from build123d import *

# Parameters (mm, degrees)
SKETCH_1_W       = 16
SKETCH_1_H       = 16
EXTRUDE_1_DEPTH  = 4
SKETCH_2_R       = 6.5
EXTRUDE_2_DEPTH  = 7
SKETCH_3_R       = 6
EXTRUDE_3_DEPTH  = 12
EXTRUDE_START    = -2
SKETCH_4_R       = 6.5
EXTRUDE_4_DEPTH  = 2
SKETCH_6_R       = 1
EXTRUDE_5_DEPTH  = 3.6
SKETCH_7_W       = 26
SKETCH_7_H       = 27
EXTRUDE_6_DEPTH  = 1.5
SKETCH_8_W       = 10
SKETCH_8_H       = 22
EXTRUDE_7_DEPTH  = 4
SKETCH_9_R       = 0.6
EXTRUDE_8_DEPTH  = 4
SKETCH_10_R      = 0.6
EXTRUDE_9_DEPTH  = 1.5
SKETCH_11_W      = 4.148660329
SKETCH_11_H      = 3.0926377
EXTRUDE_10_DEPTH = 1.5


with BuildPart() as part:
    # 草图1 → 凸台-拉伸1 (new body)
    with BuildSketch(Plane.XY):
        Rectangle(SKETCH_1_W, SKETCH_1_H)
    extrude(amount=EXTRUDE_1_DEPTH)

    # 草图2 → 凸台-拉伸2 (add)
    with BuildSketch(Plane.XY.offset(4)):
        with Locations(Location((0, 0, 0), (0, 0, 180))):
            Circle(SKETCH_2_R)
    extrude(amount=EXTRUDE_2_DEPTH)

    # 草图3 → 凸台-拉伸3 (add)
    with BuildSketch(Plane.XY.offset(11)):
        Circle(SKETCH_3_R)
    extrude(amount=EXTRUDE_3_DEPTH)

    # 草图4 → 凸台-拉伸4 (add)
    with BuildSketch(Plane.XY.offset(23).offset(EXTRUDE_START)):
        with Locations(Location((0, 0, 0), (0, 0, 180))):
            Circle(SKETCH_4_R)
    extrude(amount=EXTRUDE_4_DEPTH)

    # 草图5 → 切除-旋转2 (revolve, cut)
    with BuildSketch(Plane.XY.offset(23)):
        with BuildLine():
            Line((0, 2), (0, -2))
            ThreePointArc((0, -2), (2, 0), (0, 2))
        make_face()
    revolve(axis=Axis((0, 2, 23), (0, -1, 0)), mode=Mode.SUBTRACT)

    # 草图6 → 凸台-拉伸5 (add)
    # profile 1 of 2: a face of its own
    with BuildSketch(Plane(origin=(0, 0, 0), x_dir=(-1, 0, 0), z_dir=(0, 0, -1))):
        with BuildLine():
            Line((-1.8, 8), (-1.8, 11.5))
            ThreePointArc((-1.8, 11.5), (0, 13.3), (1.8, 11.5))
            Line((1.8, 11.5), (1.8, 8))
            Line((1.8, 8), (-1.8, 8))
        make_face()
        with Locations((0, 11.5)):
            Circle(SKETCH_6_R, mode=Mode.SUBTRACT)
    # profile 2 of 2: a face of its own
    with BuildSketch(Plane(origin=(0, 0, 0), x_dir=(-1, 0, 0), z_dir=(0, 0, -1))):
        with BuildLine():
            Line((-1.8, -8), (1.8, -8))
            Line((1.8, -8), (1.8, -11.5))
            ThreePointArc((1.8, -11.5), (0, -13.3), (-1.8, -11.5))
            Line((-1.8, -11.5), (-1.8, -8))
        make_face()
        with Locations(Location((0, -11.5, 0), (0, 0, 180))):
            Circle(SKETCH_6_R, mode=Mode.SUBTRACT)
    extrude(amount=-EXTRUDE_5_DEPTH)

    # 草图7 → 凸台-拉伸6 (add)
    with BuildSketch(Plane(origin=(0, 0, 0), x_dir=(-1, 0, 0), z_dir=(0, 0, -1))):
        with Locations((4, 0)):
            Rectangle(SKETCH_7_W, SKETCH_7_H)
    extrude(amount=EXTRUDE_6_DEPTH)

    # 草图8 → 凸台-拉伸7 (add)
    with BuildSketch(Plane(origin=(0, 0, -1.5), x_dir=(-1, 0, 0), z_dir=(0, 0, -1))):
        with Locations((16, 0)):
            Rectangle(SKETCH_8_W, SKETCH_8_H)
    extrude(amount=EXTRUDE_7_DEPTH)

    # 草图9 → 凸台-拉伸8 (add)
    with BuildSketch(Plane.ZY.offset(21)):
        with Locations(Location((-3.5, 0, 0), (0, 0, 180))):
            Circle(SKETCH_9_R)
        with Locations(Location((-3.5, 3, 0), (0, 0, 180))):
            Circle(SKETCH_9_R)
        with Locations(Location((-3.5, 6, 0), (0, 0, 180))):
            Circle(SKETCH_9_R)
        with Locations(Location((-3.5, 9, 0), (0, 0, 180))):
            Circle(SKETCH_9_R)
        with Locations(Location((-3.5, -9, 0), (0, 0, 180))):
            Circle(SKETCH_9_R)
        with Locations(Location((-3.5, -6, 0), (0, 0, 180))):
            Circle(SKETCH_9_R)
        with Locations(Location((-3.5, -3, 0), (0, 0, 180))):
            Circle(SKETCH_9_R)
    extrude(amount=EXTRUDE_8_DEPTH)

    # 草图10 → 凸台-拉伸9 (add)
    with BuildSketch(Plane.XY):
        with Locations(Location((-12, 9, 0), (0, 0, 180))):
            Circle(SKETCH_10_R)
        with Locations(Location((-15, 9, 0), (0, 0, 180))):
            Circle(SKETCH_10_R)
        with Locations(Location((-15, 6, 0), (0, 0, 180))):
            Circle(SKETCH_10_R)
        with Locations(Location((-15, 3, 0), (0, 0, 180))):
            Circle(SKETCH_10_R)
        with Locations(Location((-15, 0, 0), (0, 0, 180))):
            Circle(SKETCH_10_R)
        with Locations(Location((-15, -3, 0), (0, 0, 180))):
            Circle(SKETCH_10_R)
        with Locations(Location((-15, -6, 0), (0, 0, 180))):
            Circle(SKETCH_10_R)
        with Locations(Location((-15, -9, 0), (0, 0, 180))):
            Circle(SKETCH_10_R)
        with Locations(Location((-12, 6, 0), (0, 0, 180))):
            Circle(SKETCH_10_R)
        with Locations(Location((-12, 3, 0), (0, 0, 180))):
            Circle(SKETCH_10_R)
        with Locations(Location((-12, 0, 0), (0, 0, 180))):
            Circle(SKETCH_10_R)
        with Locations(Location((-12, -3, 0), (0, 0, 180))):
            Circle(SKETCH_10_R)
        with Locations(Location((-12, -6, 0), (0, 0, 180))):
            Circle(SKETCH_10_R)
        with Locations(Location((-12, -9, 0), (0, 0, 180))):
            Circle(SKETCH_10_R)
    extrude(amount=EXTRUDE_9_DEPTH)

    # 草图11 → 凸台-拉伸10 (add)
    with BuildSketch(Plane.XY):
        with Locations((-6.793116996, -10.371650821)):
            Rectangle(SKETCH_11_W, SKETCH_11_H)
    extrude(amount=EXTRUDE_10_DEPTH)


solid = part.part
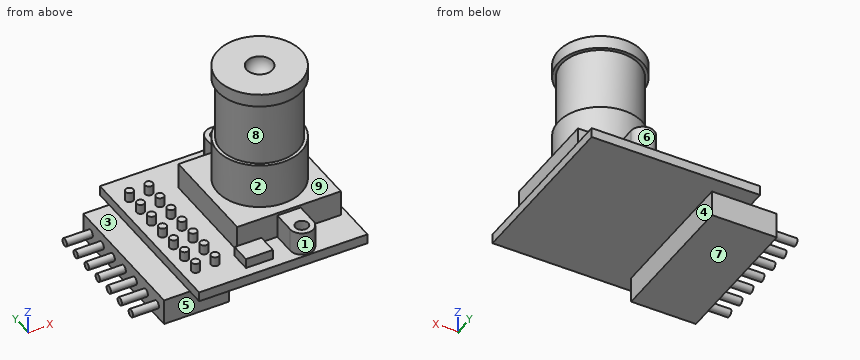
Part model, mm, in its own coordinate system. Face numbers are marked on the shaded views. A direction names the side the tool comes from. Give positions to 0.01 mm unless a question says otherwise; leave off trailing zeros. Order: outer loops, then holes, each group sorted by start corner. A loop starts at its lowest first (then second) coordinate and runs counter-clockwise, first axis right, second up. Notation, with made-up numbers: (53.5, 61) -> (70.5, 61) arc R21 ccw to (70.5, 84) -> close; hole circle Ø3 at (37, 35). An arc over 180 degrees is marked (long way). Use one line per item in the form item = value.
(1) Tool access for the marked faces 1, 2, 3, 4 and 5: list every direction of +Z, -Z, +X, -X, +Y, -Y with a clear straight run to the whole face (end or side of a thin tool).
Solution:
face_1 = +Z, -Y
face_2 = +Z
face_3 = +Z, -X, +Y, -Y
face_4 = -Z, +X, +Y, -Y
face_5 = -Z, +X, -X, -Y
(2) Flat gauge pins, fed straight in: P1, Ø1, axis at x = -12, y = 6, coming from the +Z side; P2, Ø1.2, axis at y = 6.5, z = -1, coming from the -X side; P3, Ø0.8, axis at y = -10.5, z = 1, coming from the -X side. Where does each tip first touch, or does it go through?
Solution:
P1 = 1.5
P2 = -21
P3 = -8.87
(3) Saw through at A-A (y = 9). Write the cut outline in (x, z).
Solution:
outline = (-25, -4.1) -> (-21, -4.1) -> (-21, -5.5) -> (-11, -5.5) -> (-11, -1.5) -> (9, -1.5) -> (9, 0) -> (1.8, 0) -> (1.8, 3.6) -> (-1.8, 3.6) -> (-1.8, 0) -> (-11.4, 0) -> (-11.4, 1.5) -> (-12.6, 1.5) -> (-12.6, 0) -> (-14.4, 0) -> (-14.4, 1.5) -> (-15.6, 1.5) -> (-15.6, 0) -> (-17, 0) -> (-17, -1.5) -> (-21, -1.5) -> (-21, -2.9) -> (-25, -2.9) -> close
(4) Pull direction Z, two halves, no side cores. Call the marked faces 6, 7, 8 and 9: +Z half, -Z half, draft (parallel to the pull), parting line (faces both ways), or undercut.
Solution:
face_6 = draft
face_7 = -Z half
face_8 = undercut
face_9 = +Z half
(5) Saw through at D-D (z = 10.5). Write the cut outline in (x, y).
Solution:
outline = circle Ø13 at (0, 0)
(6) Drill centre lines: line 1 (Y direction, x = 0, z = 2.25); line 2 (X direction, y = -11.5, z = 2.15); line 3 (Z direction, x = -1, y = 9). Where is each one in solid material? Low to high. Write a range as from..to.
Solution:
line_1 = -13.3..-12.5, -10.5..10.5, 12.5..13.3
line_2 = -1.8..-1, 1..1.8
line_3 = -1.5..3.6
(7) Saw through at B-B (z = 2.5). Write the cut outline in (x, y).
Solution:
outline = (-8, -8) -> (-1.8, -8) -> (-1.8, -11.5) arc R1.8 ccw to (1.8, -11.5) -> (1.8, -8) -> (8, -8) -> (8, 8) -> (1.8, 8) -> (1.8, 11.5) arc R1.8 ccw to (-1.8, 11.5) -> (-1.8, 8) -> (-8, 8) -> close; hole circle Ø2 at (0, -11.5); hole circle Ø2 at (0, 11.5)
